Here's the drawing with two shaded views (mm, measured from the low corner). I have some questions. A direction names the side the tool comes from. Round coordinates to 2 decimals unless told otherwise and drop trailing zeros. Order: outer loops, then holes, each group sorted by start corner. A loop starts at its lowest first (then second) coordinate and runs counter-clockwise, first axis right, second up.
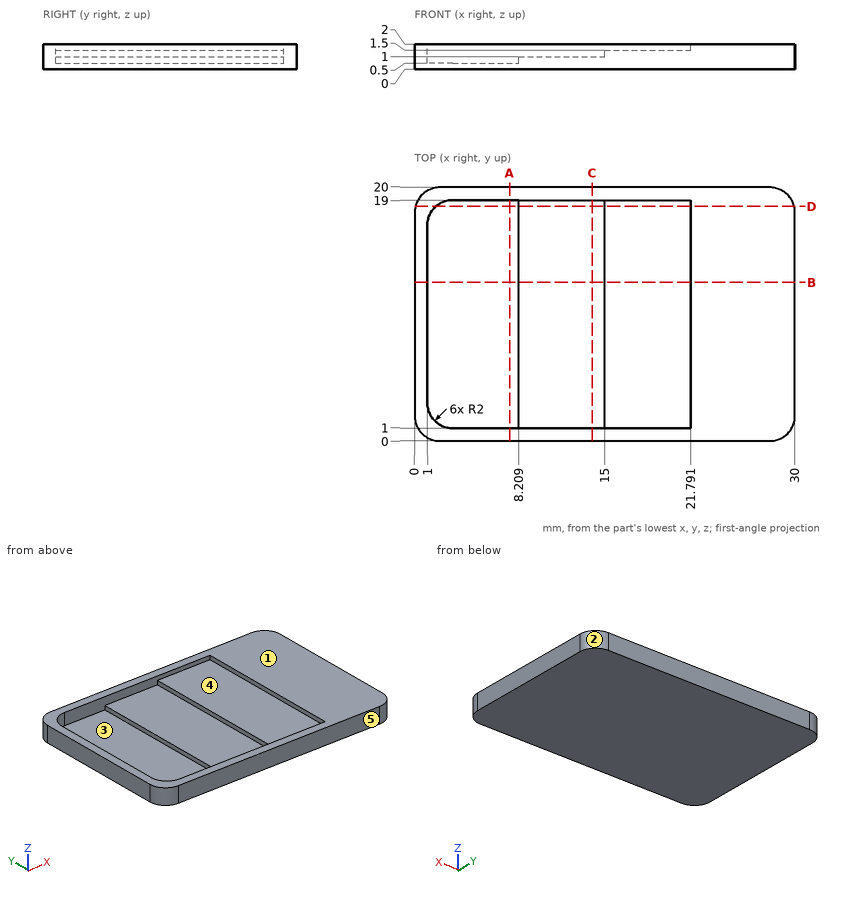
Q1. Imagine slicing it at B-B, the plane y = 12.5. Please give me the cut outline in (x, z), then the cut area to 3 significant figures.
Q2. For the marked faces 4 and 5, which set-ups out of +Z, -Z, +X, -X, +Y, -Y let a thin tool reach every point of the face, with its end or its side?
Q3. Imagine slicing it at A-A, the plane x = 7.5. Please give me the cut outline in (y, z), then the cut area to 3 significant figures.
Q4. For P1, Ø4, axis at x = 22.5, y = 18, coming from the -Z side; P2, Ø5.5, axis at x = 10, y = 9.5, coming from the +Z side, each with a flat end and sliding along its axis, tell me the tip position at first contact or that it passes through.
Q5. We'd pull the mould along X, two halves only. Please class the marked faces 1, 2 and 3: released by +X, released by -X, zero draft, split by the parting line, or undercut.
Q6. Imagine slicing it at D-D, the plane y = 18.5. Please give me the cut outline in (x, z).
Q7. I need wall thicknesses on L1, parallel to X at y = 16.5, z = 1.05; L2, parallel to Y at x = 6, z = 0.6; L3, parallel to X at y = 16.5, z = 0.95. Which ranges of each line are inside material? Lowest first, please.
Q8. Imagine slicing it at C-C, the plane x = 14. Please give me the cut outline in (y, z), then the cut area to 3 significant figures.
Filled in:
1. outline: (0, 0) - (30, 0) - (30, 2) - (21.79, 2) - (21.79, 1.5) - (15, 1.5) - (15, 1) - (8.21, 1) - (8.21, 0.5) - (1, 0.5) - (1, 2) - (0, 2) - close
1. area: 39.0 mm2
2. face 4: +Z
2. face 5: +Z, -Z, +X, -X, -Y
3. outline: (0, 0) - (20, 0) - (20, 2) - (19, 2) - (19, 0.5) - (1, 0.5) - (1, 2) - (0, 2) - close
3. area: 13.0 mm2
4. P1: stops at z = 0
4. P2: stops at z = 1
5. face 1: zero draft
5. face 2: released by +X
5. face 3: undercut
6. outline: (0.06, 0) - (29.94, 0) - (29.94, 2) - (21.79, 2) - (21.79, 1.5) - (15, 1.5) - (15, 1) - (8.21, 1) - (8.21, 0.5) - (1.68, 0.5) - (1.68, 2) - (0.06, 2) - close
7. L1: x = 0 to 1, 15 to 30
7. L2: y = 0 to 1, 19 to 20
7. L3: x = 0 to 1, 8.21 to 30
8. outline: (0, 0) - (20, 0) - (20, 2) - (19, 2) - (19, 1) - (1, 1) - (1, 2) - (0, 2) - close
8. area: 22.0 mm2
